Check sheet for the modelled part. Datum: model origin and axes. Units: mm. Round coordinates to 2 decimals unless told otherwise and drop trailing zeros. Write each loop counter-clockwise with the first axis right and the second up, starting at its lowest first coordinate (ties: lowest second). Pieces come first, ordered by that corner, then holes. Notation, with made-up numbers: (-11, 83) - (-6, 83) arc R15 ccw to (-6, 95) - close; hole circle Ø4 at (31.25, -17). An arc over 180 degrees is marked (long way). Answer as a JSON object with one key per item and string values. Group by question number.
Item 1: Thickness scan on line 1 (Z direction, x = -0.75, y = -5.5); line 2 (Y direction, x = 0.25, z = 20); line 3 (X direction, y = -0.5, z = 46). Record the ranges inside material, lowest first.
Item 2: Sectioned sample at A-A on z = 6. Record the boundary of the cut face in (x, y).
Item 3: Gauge pin test, flat ends, axial feed: P1, Ø1.5, axis at x = 2, z = 107, coming from the -Y side; P2, Ø8, axis at y = 0, z = 43, coming from the -X side; P3, Ø3, axis at x = -6, y = 1, coming from the -Z side. Record the tip position at first contact, or that the pin passes through.
```python
from build123d import *

# Parameters (mm, degrees)
IZIM1_R                     = 5
Y_KSEKLIK_EKSTR_ZYON1_DEPTH = 150
IZIM2_R                     = 7.5
Y_KSEKLIK_EKSTR_ZYON2_DEPTH = 5
RADYUS5_R                   = 5
Y_KSEKLIK_EKSTR_ZYON3_START = 5
IZIM3_R                     = 7.5
Y_KSEKLIK_EKSTR_ZYON3_DEPTH = 5
RADYUS6_R                   = 5


with BuildPart() as part:
    # Çizim1 → Yükseklik-Ekstrüzyon1 (new body)
    with BuildSketch(Plane.XY):
        Circle(IZIM1_R)
    extrude(amount=Y_KSEKLIK_EKSTR_ZYON1_DEPTH)

    # Çizim2 → Yükseklik-Ekstrüzyon2 (add)
    with BuildSketch(Plane.XY.offset(150)):
        Circle(IZIM2_R)
    extrude(amount=Y_KSEKLIK_EKSTR_ZYON2_DEPTH)

    # Radyus5
    radyus5_edges = [part.edges().sort_by_distance(p)[0] for p in [
        (-7.5, 0, 155),
    ]]
    fillet(radyus5_edges, radius=RADYUS5_R - 0.0001)  # a hair under: the kernel refuses the full size

    # Çizim3 → Yükseklik-Ekstrüzyon3 (add)
    with BuildSketch(Plane(origin=(0, 0, 0), x_dir=(-1, 0, 0), z_dir=(0, 0, -1)).offset(Y_KSEKLIK_EKSTR_ZYON3_START)):
        Circle(IZIM3_R)
    extrude(amount=-Y_KSEKLIK_EKSTR_ZYON3_DEPTH)

    # Radyus6
    radyus6_edges = [part.edges().sort_by_distance(p)[0] for p in [
        (7.5, 0, -5),
    ]]
    fillet(radyus6_edges, radius=RADYUS6_R - 0.0001)  # a hair under: the kernel refuses the full size


solid = part.part
```
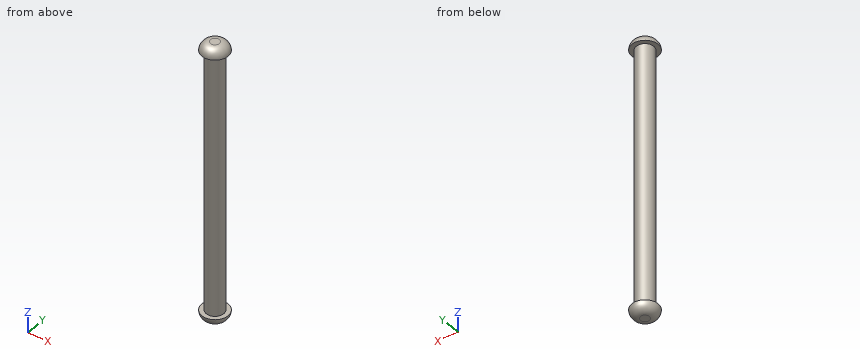
Completed:
{
 "1": {"line 1": "-3.96 to 0, 150 to 153.96", "line 2": "-4.99 to 4.99", "line 3": "-4.97 to 4.97"},
 "2": {"outline": "circle Ø10 at (0, 0)"},
 "3": {"P1": "y = -4.84", "P2": "x = -5", "P3": "z = -4.55"}
}
